Geometry: see drawing. Coordinates: mm, zero at the bounding-box minimum. A direction names the side the tool comes from. Round coordinates to 2 decimals unless told otherwise and drop trailing zeros. Loops run counter-clockwise (first coordinate to the right, second up) from the corner with the lowest first, then second, coordinate; pieces in that order, holes last.
(1) Set-up query: the marked faces 1 and 2. Return all of +Z, -Z, +X, -X, +Y, -Y with unobstructed straight access to the full face (end or side cutting, diameter ignored); none if empty.
(2) Mould query, pull axis Y, two halves, no side actions, for the marked faces 3, 4 and 5. Classes: pulls with the +Y half, pulls with the -Y half, needs draft (parallel to the pull), parting line crosses it, or undercut.
(3) Material intervals for probe 1 along Z at (x, y) = (25, 3.4); probe 2 along X at (y, z) = (1.65, 37.5); probe 3 along Z at (x, y) = (10.75, 20), sorted ascending.
(4) Section C-C, the plane y = 2.5. Return the cut outline in (x, z), plus the area to 3 significant figures.
(5) Section A-A, the plane z = 37.5. Return the cut outline in (x, y), plus the area to 3 significant figures.
(6) First-contact query: pin 1 Ø5 at (x, z) = (25, 37.5) entering from +Y. Flat tip, straight axial feed; report the tip coordinate or a pass-through.
(7) Section B-B, the plane x = 15. Return the cut outline in (y, z).
(8) Section D-D, the plane y = 15. Return the cut outline in (x, z), plus the area to 3 significant figures.
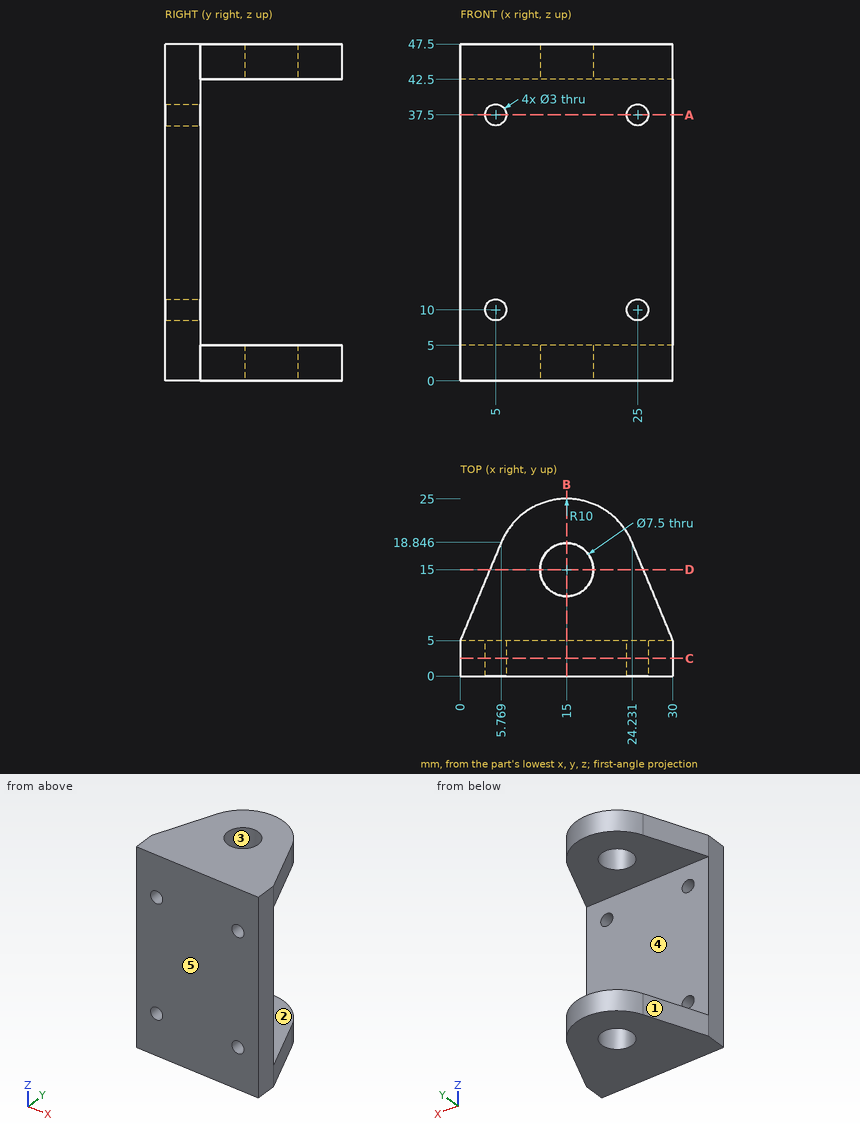
Output values:
1. face 1: +Z, -Z, -X, +Y
1. face 2: +X, -X, +Y
2. face 3: undercut
2. face 4: pulls with the +Y half
2. face 5: pulls with the -Y half
3. probe 1: z = 0 to 8.5, 11.5 to 36, 39 to 47.5
3. probe 2: x = 0 to 3.5, 6.5 to 23.5, 26.5 to 30
3. probe 3: z = 0 to 5, 42.5 to 47.5
4. outline: (0, 0) - (30, 0) - (30, 47.5) - (0, 47.5) - close; hole circle Ø3 at (5, 10); hole circle Ø3 at (5, 37.5); hole circle Ø3 at (25, 10); hole circle Ø3 at (25, 37.5)
4. area: 1,400 mm2
5. outline: (0, 0) - (3.5, 0) - (3.5, 5) - (0, 5) - close; (6.5, 0) - (23.5, 0) - (23.5, 5) - (6.5, 5) - close; (26.5, 0) - (30, 0) - (30, 5) - (26.5, 5) - close
5. area: 120 mm2
6. pin 1: stops at y = 5
7. outline: (0, 0) - (11.25, 0) - (11.25, 5) - (5, 5) - (5, 42.5) - (11.25, 42.5) - (11.25, 47.5) - (0, 47.5) - close; (18.75, 0) - (25, 0) - (25, 5) - (18.75, 5) - close; (18.75, 42.5) - (25, 42.5) - (25, 47.5) - (18.75, 47.5) - close
8. outline: (4.17, 0) - (11.25, 0) - (11.25, 5) - (4.17, 5) - close; (4.17, 42.5) - (11.25, 42.5) - (11.25, 47.5) - (4.17, 47.5) - close; (18.75, 0) - (25.83, 0) - (25.83, 5) - (18.75, 5) - close; (18.75, 42.5) - (25.83, 42.5) - (25.83, 47.5) - (18.75, 47.5) - close
8. area: 142 mm2
